from build123d import *

# Parameters (mm, degrees)
ESQUISSE4_W                  = 18.656759262
ESQUISSE4_H                  = 11.470185
ENL_V_MAT_EXTRU_1_DEPTH      = 10
ENL_V_MAT_EXTRU_1_DEPTH_BACK = 10
ESQUISSE5_R                  = 12.05
ESQUISSE5_R_2                = 11.9
BOSS_EXTRU_1_DEPTH           = 13
ESQUISSE6_R                  = 1.5
ENL_V_MAT_EXTRU_2_DEPTH      = 5
R_P_TITION_CIRCULAIRE1_COUNT = 3


with BuildPart() as part:
    # Esquisse1 → R_volution1 (revolve)
    with BuildSketch(Plane.XY):
        Polygon((-30, 0), (-30, 17), (0, 17), (0, 18.4), (22, 18.4), (22, 0), align=None)
    revolve(axis=Axis((-59.117838542, 0, 0), (1, 0, 0)))

    # Esquisse3 → R_volution2 (revolve)
    with BuildSketch(Plane.XY):
        Polygon((22, -1), (28.5, -1), (28.5, -4), (44, -4), (44, -7), (22, -7), align=None)
    revolve(axis=Axis((8.410725031, -7, 0), (1, 0, 0)))

    # Esquisse4 → Enl_v. mat.-Extru.1 (cut, two sides)
    with BuildSketch(Plane.XY) as enl_v_mat_extru_1_sk:
        with Locations((41.328379631, 1.1350925)):
            Rectangle(ESQUISSE4_W, ESQUISSE4_H)
    extrude(amount=ENL_V_MAT_EXTRU_1_DEPTH, mode=Mode.SUBTRACT)
    extrude(enl_v_mat_extru_1_sk.sketch, amount=-ENL_V_MAT_EXTRU_1_DEPTH_BACK, mode=Mode.SUBTRACT)

    # Esquisse5 → Boss.-Extru.1 (add)
    with BuildSketch(Plane.ZY.offset(30)):
        Circle(ESQUISSE5_R)
        Circle(ESQUISSE5_R_2, mode=Mode.SUBTRACT)
    extrude(amount=BOSS_EXTRU_1_DEPTH)

    # Esquisse6 → Enl_v. mat.-Extru.2 (cut)
    with BuildSketch(Plane(origin=(22, 0, 0), x_dir=(0, 0, -1), z_dir=(1, 0, 0))):
        with Locations((0, 15.5)):
            Circle(ESQUISSE6_R)
        with Locations((7.75, 13.423393759)):
            Circle(ESQUISSE6_R)
        with Locations((-7.75, 13.423393759)):
            Circle(ESQUISSE6_R)
    enl_v_mat_extru_2 = extrude(amount=-ENL_V_MAT_EXTRU_2_DEPTH, mode=Mode.SUBTRACT)

    # R_p_tition circulaire1: Enl_v. mat.-Extru.2 ×3 about axis
    r_p_tition_circulaire1_axis = Axis((0, 0, 0), (1, 0, 0))
    for i in range(1, R_P_TITION_CIRCULAIRE1_COUNT):
        add(enl_v_mat_extru_2.rotate(r_p_tition_circulaire1_axis, i * 360 / R_P_TITION_CIRCULAIRE1_COUNT), mode=Mode.SUBTRACT)


solid = part.part
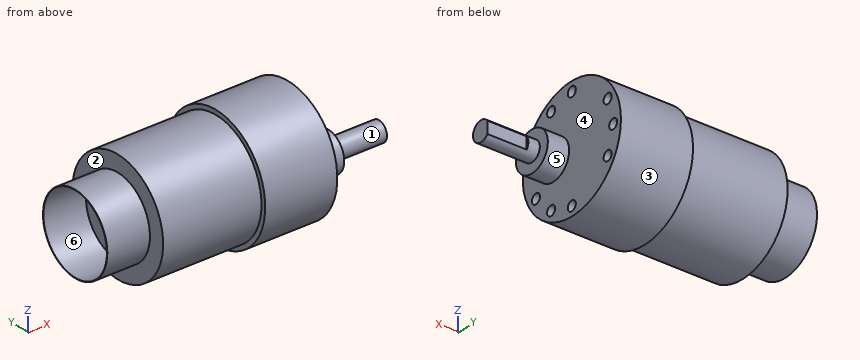
For this review, take the finished solid that the model builds, in its own axes (mm). Face numbers are marked on the shaded views. A direction names the side the tool comes from. Round coordinates to 2 decimals unless told otherwise and drop trailing zeros. Loops run counter-clockwise (first coordinate to the right, second up) from the corner with the lowest first, then second, coordinate; pieces in that order, holes last. Notation, with made-up numbers: (57.5, -24.75) - (100.5, -24.75) arc R22 ccw to (100.5, -1.75) - close; hole circle Ø9 at (77.25, -10). An arc over 180 degrees is marked (long way). Put each result on its own line as item: value. Start each with the question number.
1. Consider section A-A on y = 0. State the section outline as (x, z) points.
2. Mouldability with a two-part tool opening along Z and no side actions: class the marked faces 4, 5 and 6 as +Z half, -Z half, draft (parallel to the pull), parting line (faces both ways), or undercut.
3. Insertion check: P1, Ø2.5, axis at y = -13.5, z = 8.5, coming from the +X side; P2, Ø1.8, axis at y = 13.42, z = -7.75, coming from the +X side; P3, Ø6, axis at x = -13.5, y = 1, coming from the -Z side; P4, Ø3, axis at y = -4, z = 12, coming from the -X side. Each pin has a flat end and moves straight along its axis. Give the tip position at first contact, or say it passes through.
4. Consider section D-D on x = -12.5. State the section outline as (y, z) points.
5. Consider section C-C on x = 18.5. State how many separate pieces and enclosed holes the cut face has, plus the area to 3 significant figures.
6. For the marked faces 1, 2 and 3, list the 3-axis set-ups (+Z, -Z, +X, -X, +Y, -Y) from which the entire face can be reached by the end or side of a thin tool; tool diameter is ignored.
7. For probe 1 along Z at (x, y) = (18, 0); probe 2 along Y at (x, z) = (18, 8); probe 3 along Y at (x, z) = (19, 7.75), list the stretches that pass through material, from the lowest coordinate up. Write a range as [from, to].
Result sheet:
1. outline: (-43, -12.05) - (-30, -12.05) - (-30, -17) - (0, -17) - (0, -18.4) - (22, -18.4) - (22, -17) - (17, -17) - (17, -14) - (22, -14) - (22, 14) - (17, 14) - (17, 17) - (22, 17) - (22, 18.4) - (0, 18.4) - (0, 17) - (-30, 17) - (-30, 12.05) - (-43, 12.05) - (-43, 11.9) - (-30, 11.9) - (-30, -11.9) - (-43, -11.9) - close
2. face 4: draft
2. face 5: parting line
2. face 6: undercut
3. P1: x = 22
3. P2: x = 17
3. P3: z = -17
3. P4: x = -43
4. outline: circle Ø34 at (0, 0)
5. separate pieces: 1
5. enclosed holes: 9
5. area: 1,000 mm^2
6. face 1: +X
6. face 2: -X
6. face 3: +X, -X
7. probe 1: [-18.4, -17], [-14, 14], [17, 18.4]
7. probe 2: [-16.57, -14.9], [-11.94, 11.94], [14.9, 16.57]
7. probe 3: [-16.69, -14.92], [-11.92, 11.92], [14.92, 16.69]
